```python
from build123d import *

# Parameters (mm, degrees)
F0_R     = 19.05
F1_DEPTH = 177.8
F2_R     = 12.7
F3_DEPTH = 177.8
F5_START = 7.112
F4_R     = 4.5268076309
F5_DEPTH = 16.51
F7_START = 6.604
F6_R     = 3.1768025879
F7_DEPTH = 17.78


with BuildPart() as f1:
    # F0 (on Front) → F1 (new body)
    with BuildSketch(Plane.XZ):
        Circle(F0_R)
    extrude(amount=F1_DEPTH)

    # F2 (on Front) → F3 (cut)
    with BuildSketch(Plane.XZ):
        Circle(F2_R)
    extrude(amount=F3_DEPTH, mode=Mode.SUBTRACT)

    # F4 (on Top) → F5 (join)
    with BuildSketch(Plane.XY.offset(F5_START)):
        with Locations((0, -91.6567370296)):
            Circle(F4_R)
    extrude(amount=F5_DEPTH)

    # F6 (on Top) → F7 (cut)
    with BuildSketch(Plane.XY.offset(F7_START)):
        with Locations((0, -91.5180891752)):
            Circle(F6_R)
    extrude(amount=F7_DEPTH, mode=Mode.SUBTRACT)


solid = f1.part
```
The model under review builds one solid part; all positions refer to its coordinate system, in mm. A direction names the side the tool comes from. Coordinates: 2 decimals unless noted, no trailing zeros. Write each loop counter-clockwise with the first axis right and the second up, starting at its lowest first coordinate (ties: lowest second). Pieces come first, ordered by that corner, then holes. Notation, with made-up numbers: (34.25, -11) - (89.25, -11) arc R32 cw to (89.25, 21) - close; hole circle Ø5 at (44, 8.25). An arc over 180 degrees is marked (long way). Answer in a Markdown table with one row per item. Add a question column.
Q1. Consider section C-C on y = -29. Give the boundary of the cut face in (x, z).
Q2. Consider section D-D on z = -7. Give the boundary of the cut face in (x, y), then the cut area to 3 significant figures.
Q3. To check wall thickness, follow line 1 along Z through (x, y) = (-0.5, -26.5); line 2 along X through (y, z) = (-89, 9.5); line 3 along X through (y, z) = (-46.5, 4). State the ranges of each line that lie inside material, in increasing order. Write a range as from..to.
Q4. Draft analysis for pull direction Z (two halves, no side actions). For faces 3 (the face through (1, -95, 23.622)), 4 (the face through (4.18, -93.39, 9.87)), 5 (the face through (1, -95, 7.112)), 6 (the face through (4, -177.8, -12.4)), state which applies: +Z half, -Z half, draft (parallel to the pull), parting line (faces both ways), or undercut.
Q5. Consider section B-B on z = 0. Give the boundary of the cut face in (x, y), then the cut area to 3 significant figures.
Q6. Consider section A-A on x = 0. Give the boundary of the cut face in (y, z).
Q7. Clearance check with flat-ended pins moving along their axes: pin 1 (1 mm diameter, centred on x = 4.5, y = -101, fed in from -Z); pin 2 (10 mm diameter, centred on x = 1.5, y = -93.5, fed in from -Z); pin 3 (1.5 mm diameter, centred on x = -11, y = -127.5, fed in from -Z); pin 4 (1.5 mm diameter, centred on x = -5, z = -12, fed in from +Y). State where each tip first meets the part, or that it passes through.
Q8. For faces 1 (the face through (-0.981, -96.076, 21.019)), 2 (the face through (4, 0, -12.4)), list the 3-axis set-ups (+Z, -Z, +X, -X, +Y, -Y) from which the entire face can be reached by the end or side of a thin tool; tool diameter is ignored.
Answers below:
| question | item | result |
|---|---|---|
| 1 | outline | circle Ø38.1 at (0, 0); hole circle Ø25.4 at (0, 0) |
| 2 | outline | (-17.72, -177.8) - (-10.6, -177.8) - (-10.6, 0) - (-17.72, 0) - close; (10.6, -177.8) - (17.72, -177.8) - (17.72, 0) - (10.6, 0) - close |
| 2 | area | 2,530 mm² |
| 3 | line 1 | -19.04..-12.69, 12.69..19.04 |
| 3 | line 2 | -16.51..-8.43, -3.67..-1.94, 1.94..3.67, 8.43..16.51 |
| 3 | line 3 | -18.63..-12.05, 12.05..18.63 |
| 4 | face 3 | +Z half |
| 4 | face 4 | undercut |
| 4 | face 5 | undercut |
| 4 | face 6 | draft |
| 5 | outline | (-19.05, -177.8) - (-12.7, -177.8) - (-12.7, 0) - (-19.05, 0) - close; (12.7, -177.8) - (19.05, -177.8) - (19.05, 0) - (12.7, 0) - close |
| 5 | area | 2,260 mm² |
| 6 | outline | (-177.8, -19.05) - (0, -19.05) - (0, -12.7) - (-177.8, -12.7) - close; (-177.8, 12.7) - (-96.18, 12.7) - (-96.18, 7.11) - (-94.69, 7.11) - (-94.69, 23.62) - (-96.18, 23.62) - (-96.18, 19.05) - (-177.8, 19.05) - close; (-88.34, 7.11) - (-87.13, 7.11) - (-87.13, 12.7) - (0, 12.7) - (0, 19.05) - (-87.13, 19.05) - (-87.13, 23.62) - (-88.34, 23.62) - close |
| 7 | pin 1 | z = -18.63 |
| 7 | pin 2 | z = -19.05 |
| 7 | pin 3 | z = -16.06 |
| 7 | pin 4 | y = 0 |
| 8 | face 1 | +Z |
| 8 | face 2 | +Z, -Z, +X, -X, +Y |
